For this review, take the finished solid that the model builds, in its own axes (mm). A direction names the side the tool comes from. Coordinates: 2 decimals unless noted, no trailing zeros. Loops run counter-clockwise (first coordinate to the right, second up) from the corner with the lowest first, then second, coordinate; pieces in that order, holes last. Notation, with made-up numbers: (-29.5, 51.5) -> (-21.5, 51.5) arc R24 ccw to (-21.5, 66.5) -> close; hole circle Ø5 at (65.25, -30.75). An arc over 180 degrees is marked (long way). One line per item, written item: value.
from build123d import *

# Parameters (mm, degrees)
SKETCH_2_W          = 12
SKETCH_2_H          = 80
EXTRUDE_1_DEPTH     = 45
FILLET_1_R          = 10
SKETCH_3_R          = 5
CUT_EXTRUDE_1_DEPTH = 62.392181913
SKETCH_5_W          = 10
SKETCH_5_H          = 26
CUT_EXTRUDE_2_DEPTH = 62.392181913
SKETCH_6_R          = 18
EXTRUDE_2_DEPTH     = 25
EXTRUDE_3_DEPTH     = 15
SKETCH_8_R          = 9
CUT_EXTRUDE_3_DEPTH = 81.311892021


with BuildPart() as part:
    # Sketch 2 → Extrude 1 (new body)
    with BuildSketch(Plane(origin=(0, 0, 0), x_dir=(0, 0, -1), z_dir=(1, 0, 0))):
        with Locations((-6, 0)):
            Rectangle(SKETCH_2_W, SKETCH_2_H)
    extrude(amount=EXTRUDE_1_DEPTH)

    # Fillet 1
    fillet_1_edges = [part.edges().sort_by_distance(p)[0] for p in [
        (45, -40, 6),
        (45, 40, 6),
    ]]
    fillet(fillet_1_edges, radius=FILLET_1_R)

    # Sketch 3 → Cut-Extrude 1 (cut, through all)
    with BuildSketch(Plane.XY.offset(12)):
        with Locations((35, 30)):
            Circle(SKETCH_3_R)
        with Locations((35, -30)):
            Circle(SKETCH_3_R)
    extrude(amount=-CUT_EXTRUDE_1_DEPTH, mode=Mode.SUBTRACT)

    # Sketch 5 → Cut-Extrude 2 (cut, through all)
    with BuildSketch(Plane(origin=(45, 0, 0), x_dir=(0, 0, -1), z_dir=(1, 0, 0))):
        Rectangle(SKETCH_5_W, SKETCH_5_H)
    extrude(amount=-CUT_EXTRUDE_2_DEPTH, mode=Mode.SUBTRACT)



with BuildPart() as body_2:
    # Sketch 6 → Extrude 2 (new body)
    with BuildSketch(Plane.ZY):
        with Locations((47, 0)):
            Circle(SKETCH_6_R)
    extrude(amount=-EXTRUDE_2_DEPTH)


with BuildPart() as part_1:
    add(part.part)

    add(body_2.part)  # Extrude 3 merges body 2
    # Sketch 7 → Extrude 3 (add)
    with BuildSketch(Plane.ZY):
        with BuildLine():
            Line((12, 40), (55.731751958, 15.740282963))
            ThreePointArc((55.731751958, 15.740282963), (65, 0), (55.731751958, -15.740282963))
            Line((55.731751958, -15.740282963), (12, -40))
            Line((12, -40), (12, 40))
        make_face()
    extrude(amount=-EXTRUDE_3_DEPTH)

    # Sketch 8 → Cut-Extrude 3 (cut, through all)
    with BuildSketch(Plane(origin=(25, 0, 0), x_dir=(0, 0, -1), z_dir=(1, 0, 0))):
        with Locations((-47, 0)):
            Circle(SKETCH_8_R)
    extrude(amount=-CUT_EXTRUDE_3_DEPTH, mode=Mode.SUBTRACT)


solid = part_1.part
1. Take a section at C-C, the plane x = 14. Give the boundary of the cut face in (y, z).
Return value:
outline: (-40, 0) -> (-13, 0) -> (-13, 5) -> (13, 5) -> (13, 0) -> (40, 0) -> (40, 12) -> (15.74, 55.73) arc R18 ccw to (-15.74, 55.73) -> (-40, 12) -> close; hole circle Ø18 at (0, 47)
2. To check wall thickness, follow probe 1 along Y at (x, z) = (35, 8.5); probe 2 along X at (y, z) = (34, 17); probe 3 along Z at (x, y) = (37.5, 20). State the ranges of each line that lie inside material, in increasing order. Write a range as from..to.
Return value:
probe 1: y = -40..-35, -25..25, 35..40
probe 2: x = 0..15
probe 3: z = 0..12
3. Take a section at D-D, the plane z = 47. Give the boundary of the cut face in (x, y).
Return value:
outline: (0, -20.58) -> (15, -20.58) -> (15, -18) -> (25, -18) -> (25, -9) -> (0, -9) -> close; (0, 9) -> (25, 9) -> (25, 18) -> (15, 18) -> (15, 20.58) -> (0, 20.58) -> close
4. The part is to be moulded in two halves that separate along Y. For faces 1 (the flat face through (7.4, -27.7, 34.17)), 2 (the flat face through (0, 1, 26)), 3 (the flat face through (23, -13, 3)), say which applies: pulls with the +Y half, pulls with the -Y half, needs draft (parallel to the pull), parting line crosses it, or undercut.
Return value:
face 1: pulls with the -Y half
face 2: needs draft
face 3: undercut
5. For faces 4 (the flat face through (15, 1, 24)), 5 (the flat face through (23, 0, 5)), 6 (the flat face through (25, 8.3, 42.7)), 7 (the cylindrical face through (30, -30, 6)), 8 (the flat face through (22, 26, 0)), list the 3-axis set-ups (+Z, -Z, +X, -X, +Y, -Y) from which the entire face can be reached by the end or side of a thin tool; tool diameter is ignored.
Return value:
face 4: +X
face 5: -Z, +X, -X
face 6: +Z, +X, +Y, -Y
face 7: +Z, -Z
face 8: -Z, +X, -X, +Y, -Y
6. Take a section at A-A, the plane x = 19.5. Give the boundary of the cut face in (y, z).
Return value:
outline: (-40, 0) -> (-13, 0) -> (-13, 5) -> (13, 5) -> (13, 0) -> (40, 0) -> (40, 12) -> (-40, 12) -> close; circle Ø36 at (0, 47); hole circle Ø18 at (0, 47)
7. Insertion check: pin 1 Ø1 at (y, z) = (11, 19.5) entering from +X; pin 2 Ø1 at (x, z) = (10, 24) entering from -Y; pin 3 Ø8 at (y, z) = (9, 28.5) entering from +X; pin 4 Ø14.5 at (y, z) = (0, 47) entering from +X. Each pin has a flat end and moves straight along its axis. Give the tip position at first contact, or say it passes through.
Return value:
pin 1: stops at x = 15
pin 2: stops at y = -33.62
pin 3: stops at x = 25
pin 4: passes through
8. Take a section at B-B, the plane y = 0. Give the boundary of the cut face in (x, z), and give its area (3 significant figures).
Return value:
outline: (0, 5) -> (45, 5) -> (45, 12) -> (15, 12) -> (15, 29) -> (25, 29) -> (25, 38) -> (0, 38) -> close; (0, 56) -> (25, 56) -> (25, 65) -> (0, 65) -> close
area: 1,020 mm2
